Model file for the job. Use its own axes, mm. Face numbers are marked on the shaded views. A direction names the side the tool comes from. Round coordinates to 2 decimals unless told otherwise and drop trailing zeros. Order: outer loops, then holes, each group sorted by start corner. A loop starts at its lowest first (then second) coordinate and runs counter-clockwise, first axis right, second up. Notation, with made-up numbers: (60.25, 81) - (67.25, 81) arc R23 cw to (67.25, 117) - close; hole circle Ø5 at (57, -33.75). An arc over 180 degrees is marked (long way). Write item = value, one per line.
```python
from build123d import *

# Parameters (mm, degrees)
SKETCH1_R           = 9.5
SKETCH1_R_2         = 5
BOSS_EXTRUDE1_DEPTH = 14.5
SKETCH2_W           = 0.167239634
SKETCH2_H           = 0.858355734
SKETCH3_R           = 9
SKETCH3_R_2         = 5.5
CUT_EXTRUDE1_DEPTH  = 0.5


with BuildPart() as part:
    # Sketch1 → Boss-Extrude1 (new body, symmetric)
    with BuildSketch(Plane.XY):
        Circle(SKETCH1_R)
        Circle(SKETCH1_R_2, mode=Mode.SUBTRACT)
    extrude(amount=BOSS_EXTRUDE1_DEPTH, both=True)

    # Sketch2 → Cut-Revolve1 (revolve, cut)
    with BuildSketch(Plane(origin=(0, 0, 0), x_dir=(1, 0, 0), z_dir=(0, 1, 0))):
        with Locations((9.416380183, -11.320822133)):
            Rectangle(SKETCH2_W, SKETCH2_H)
        with Locations((9.416380183, 11.320822133)):
            Rectangle(SKETCH2_W, SKETCH2_H)
    revolve(axis=Axis((0, 0, 0), (0, 0, 1)), mode=Mode.SUBTRACT)

    # Sketch3 → Cut-Extrude1 (cut)
    with BuildSketch(Plane.XY.offset(14.5)):
        Circle(SKETCH3_R)
        Circle(SKETCH3_R_2, mode=Mode.SUBTRACT)
    cut_extrude1 = extrude(amount=-CUT_EXTRUDE1_DEPTH, mode=Mode.SUBTRACT)

    # Mirror1: Cut-Extrude1 across plane
    add(cut_extrude1.mirror(Plane.XY), mode=Mode.SUBTRACT)


solid = part.part
```
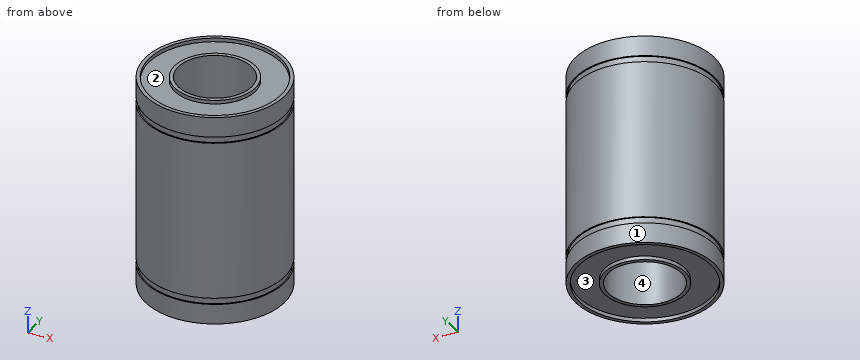
1) Cut at A-A (z = -8.25). Write the cut outline in (x, y).
Conclusion:
outline = circle Ø19 at (0, 0); hole circle Ø10 at (0, 0)
2) 3-axis set-ups, long thin cutter, end or side, ignore diameter. For the marked faces 3 and 4: which of +Z, -Z, +X, -X, +Y, -Y reach the whole face in a straight line?
Conclusion:
face_3 = -Z
face_4 = +Z, -Z
3) Flat gauge pins, fed straight in: pin 1 Ø5 at (x, z) = (5.5, 10.5) entering from +Y; pin 2 Ø1.5 at (x, z) = (4.5, -4) entering from -Y; pin 3 Ø3 at (y, z) = (-4, -1) entering from +X. Where does each tip first touch, or does it go through?
Conclusion:
pin_1 = 9.01
pin_2 = -8.73
pin_3 = 9.17
4) Wall check: line 1 along Y through (x, z) = (0, -14.15); line 2 along Y through (x, z) = (0, -8.25); line 3 along Z through (x, y) = (3, -7.5). Give the ranges that are in metal, low to high.
Conclusion:
line_1 = -9.5 to -9, -5.5 to -5, 5 to 5.5, 9 to 9.5
line_2 = -9.5 to -5, 5 to 9.5
line_3 = -14 to 14
5) Mould opens along X. For the marked faces 1 and 2 say: +X half, -X half, draft (parallel to the pull), parting line (faces both ways), or undercut.
Conclusion:
face_1 = parting line
face_2 = undercut
